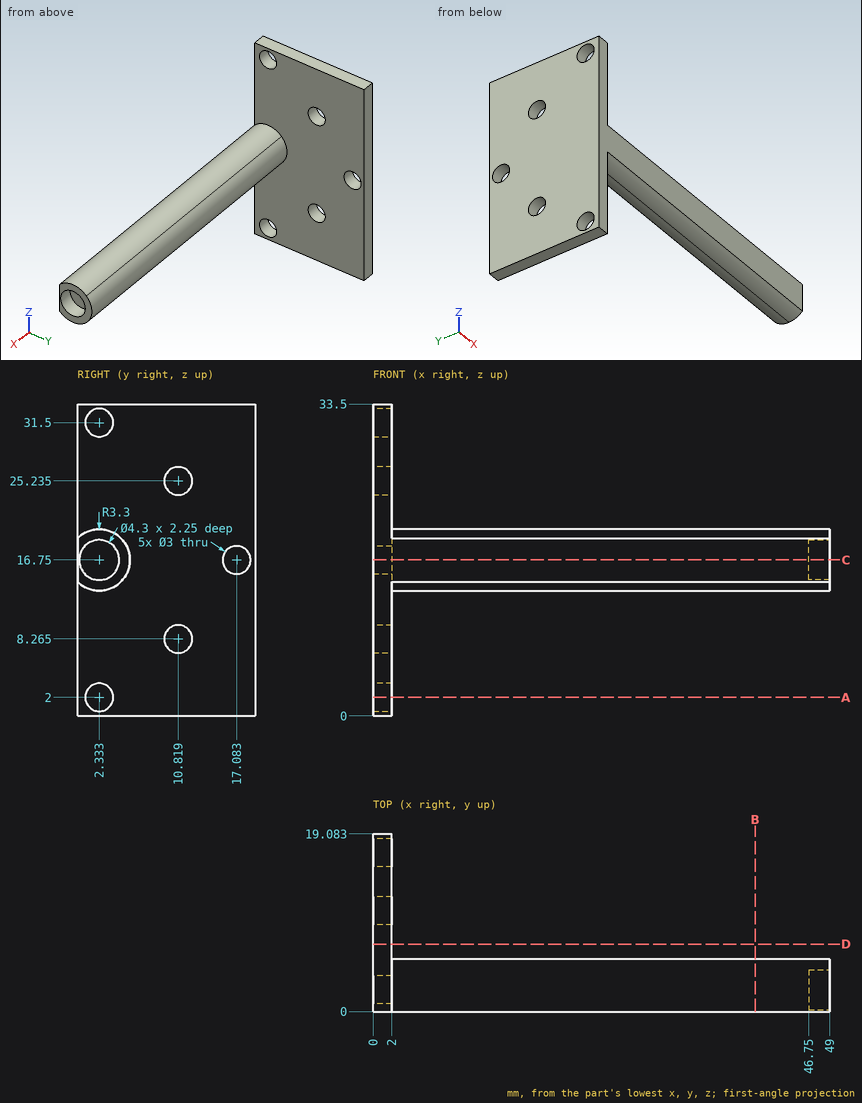
Could you check a few things on this drawing? It's one solid part, dimensions in mm from its lowest x, y, z. Give positions to 0.01 mm unless a question says otherwise; leave off trailing zeros. Loops run counter-clockwise (first coordinate to the right, second up) from the corner with the lowest first, then second, coordinate; pieces in that order, holes last. Notation, with made-up numbers: M 82,-3.5 L 106,-3.5 A19 ccw 106,32.5 Z; hole C 57.25,7.25 d1. An arc over 180 degrees is marked long. Return JSON: item names as keys, results as strings.
Item 1: Imagine slicing it at D-D on y = 7.25. List the corners of the cut face in (x, z) for me.
A:
{"outline": "M 0,0 L 2,0 L 2,33.5 L 0,33.5 Z"}
Item 2: Please list where these lines run through material, in increasing order: line 1 (Y direction, x = 1.5, z = 16.75); line 2 (Y direction, x = 48.3, z = 16.75); line 3 (X direction, y = 15, z = 31.5).
A:
{"line 1": "y = 0 to 15.58, 18.58 to 19.08", "line 2": "y = 0 to 0.18, 4.48 to 5.63", "line 3": "x = 0 to 2"}
Item 3: I'm going to push flat-ended pins straight in: pin 1 Ø1.3 at (y, z) = (3, 17.5) entering from +X; pin 2 Ø3.5 at (y, z) = (10.82, 8.26) entering from -X; pin 3 Ø9.5 at (y, z) = (9, 24.5) entering from +X. Where does each tip first touch, or does it pass through?
A:
{"pin 1": "stops at x = 46.75", "pin 2": "stops at x = 0", "pin 3": "stops at x = 2"}
Item 4: Imagine slicing it at C-C on z = 16.75. List the corners of the cut face in (x, y) for me, then the cut area to 3 significant figures.
A:
{"outline": "M 0,0 L 49,0 L 49,0.18 L 46.75,0.18 L 46.75,4.48 L 49,4.48 L 49,5.63 L 2,5.63 L 2,15.58 L 0,15.58 Z; M 0,18.58 L 2,18.58 L 2,19.08 L 0,19.08 Z", "area": "287 mm^2"}
Item 5: Imagine slicing it at A-A on z = 2. List the corners of the cut face in (x, y) for me.
A:
{"outline": "M 0,0 L 2,0 L 2,0.83 L 0,0.83 Z; M 0,3.83 L 2,3.83 L 2,19.08 L 0,19.08 Z"}
Item 6: Imagine slicing it at B-B on x = 41. List the corners of the cut face in (y, z) for me, then the cut area to 3 significant figures.
A:
{"outline": "M 0,14.42 A3.3 ccw long 0,19.08 Z", "area": "31.1 mm^2"}
